Autodesk Fusion 360 part; units mm, degrees
sketch "Sketch1" plane through (0, 0, 0) normal (0, 0, 1) x (1, 0, 0)
  line L0 (0, 0) -> (20, 0)
  line L1 (20, 0) -> (20, 40.5)
  line L2 (20, 40.5) -> (0, 40.5)
  line L3 (0, 40.5) -> (0, 0)
  line L4 (10, 40.5) -> (10, 0) construction
  circle A0 centre (2.8, 37.7) radius 1.5
  circle A1 centre (2.8, 2.8) radius 1.5
  circle A2 centre (17.2, 37.7) radius 1.5
  circle A3 centre (17.2, 2.8) radius 1.5
  dimension "d1" = 20
  dimension "d2" = 40.5
  dimension "d3" = 3
  dimension "d4" = 3
  dimension "d5" = 2.8
  dimension "d6" = 2.8
  dimension "d7" = 2.8
  dimension "d8" = 2.8
extrude "Extrude1" add sketch "Sketch1" along normal blind 1.6
fillet "Fillet1" radius 1.5 4 edges at (20, 0, 0.8) (20, 40.5, 0.8) (0, 40.5, 0.8) (0, 0, 0.8)
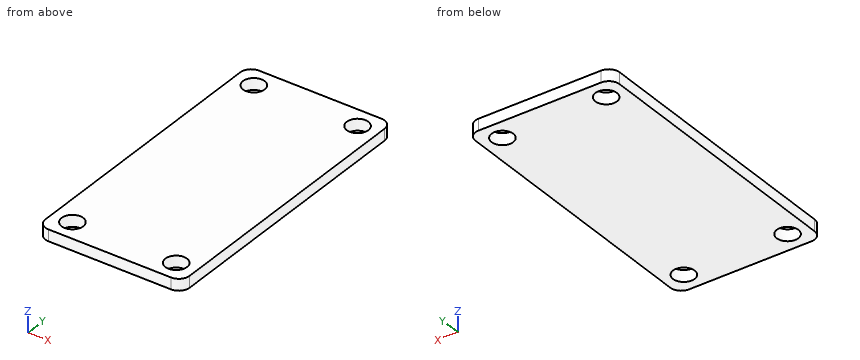
Read the model definition and answer for the solid it produces. Units are mm, in the model's axes. Give positions to 0.01 mm unless a question says otherwise; leave off trailing zeros. Write each loop counter-clockwise with the first axis right and the second up, starting at its lowest first coordinate (ties: lowest second). Pieces come first, ordered by that corner, then holes. Notation, with made-up numbers: (37, 42) - (53, 42) arc R11 cw to (53, 46) - close; hole circle Ø6 at (46.25, -6.5). An arc over 180 degrees is marked (long way). Use CSV: the item, a comma, the result in double quotes. Start each with the question number.
Item 1: The part is cut by section C-C, the plane z = 0.3. Give the vertices of the cut face in (x, y), and give its area (3 significant figures).
Item 2: Consider line 1 (Y direction, x = 2.8, z = 0.9); line 2 (X direction, y = 38.5, z = 0.55); line 3 (Y direction, x = 19, z = 0.3). Determine where each line is inside the solid, lowest interval first.
Item 3: A flat-ended cylindrical pin translates along its axis: P1, Ø3.5, axis at x = 2.8, y = 37.7, coming from the -Z side. Find the tip coordinate at first contact, or state that the pin passes through.
Item 4: The part is cut by section A-A, the plane x = 17.2. Give the vertices of the cut face in (y, z).
Item 5: The part is cut by section B-B, the plane y = 2.8. Give the vertices of the cut face in (x, z), and give its area (3 significant figures).
Taken from the geometry:
1,outline,"(0, 1.5) arc R1.5 ccw to (1.5, 0) - (18.5, 0) arc R1.5 ccw to (20, 1.5) - (20, 39) arc R1.5 ccw to (18.5, 40.5) - (1.5, 40.5) arc R1.5 ccw to (0, 39) - close; hole circle Ø3 at (2.8, 2.8); hole circle Ø3 at (2.8, 37.7); hole circle Ø3 at (17.2, 2.8); hole circle Ø3 at (17.2, 37.7)"
1,area,"780 mm2"
2,line 1,"0 to 1.3, 4.3 to 36.2, 39.2 to 40.5"
2,line 2,"0 to 1.53, 4.07 to 15.93, 18.47 to 20"
2,line 3,"0.09 to 40.41"
3,P1,"z = 0"
4,outline,"(0, 0) - (1.3, 0) - (1.3, 1.6) - (0, 1.6) - close; (4.3, 0) - (36.2, 0) - (36.2, 1.6) - (4.3, 1.6) - close; (39.2, 0) - (40.5, 0) - (40.5, 1.6) - (39.2, 1.6) - close"
5,outline,"(0, 0) - (1.3, 0) - (1.3, 1.6) - (0, 1.6) - close; (4.3, 0) - (15.7, 0) - (15.7, 1.6) - (4.3, 1.6) - close; (18.7, 0) - (20, 0) - (20, 1.6) - (18.7, 1.6) - close"
5,area,"22.4 mm2"
